Input: part model. Units: mm. Frame: model coordinates. A direction names the side the tool comes from. Round coordinates to 2 decimals unless told otherwise and drop trailing zeros. Loops run counter-clockwise (first coordinate to the right, second up) from the corner with the lowest first, then second, coordinate; pieces in that order, holes last. Notation, with made-up numbers: (83, -15) - (97, -15) arc R21 cw to (97, 19) - close; hole circle Ø3 at (87, 64). An arc over 180 degrees is marked (long way). One line per question, with ' | ' between items. Start each with the question number.
Item 1: Set-up query: faces 1 (the face through (-24.03, -24.06, 39.22)), 2 (the face through (-13, -20, 24.5)), 3 (the face through (-14.24, -24, 5.39)), 4 (the face through (-3, -24, 34.243)), 5 (the face through (-3, -20, 29.5)). Return all of +Z, -Z, +X, -X, +Y, -Y with unobstructed straight access to the full face (end or side cutting, diameter ignored); none if empty.
Item 2: Section A-A, the plane z = 6.5. Return loops of the section in (x, y), plus the area to 3 significant figures.
Item 3: Section B-B, the plane z = 29. Return loops of the section in (x, y), plus the area to 3 significant figures.
Item 4: Draft query along Y for faces 6 (the face through (-20, -24, 0)), 7 (the face through (-23.686, -29.719, 19.975)), 8 (the face through (-23, -28, 29.5)), 9 (the face through (-23, -20, 29.5)). Return one class per face: pulls with the +Y half, pulls with the -Y half, needs draft (parallel to the pull), parting line crosses it, or undercut.
Item 5: First-contact query: pin 1 (0.6 mm diameter, centred on x = -23, y = -28.5, fed in from +Z); pin 2 (1.8 mm diameter, centred on x = -13.23, z = 34.24, fed in from -Y); pin 3 (0.7 mm diameter, centred on x = -3, y = -25, fed in from -Z); pin 4 (5 mm diameter, centred on x = -13.23, z = 6.5, fed in from +Y). Flat tips, straight axial feed; report the tip coordinate or a pass-through.
Item 6: Section D-D, the plane z = 22.5. Return loops of the section in (x, y), plus the area to 3 significant figures.
Item 7: Section C-C, the plane y = -23.5. Give the number of separate pieces and of enclosed holes in the cut face, plus the area to 3 significant figures.
Item 8: Material intervals for line 1 along Y through (x, z) = (-21, 39.5); line 2 along Z through (x, y) = (-12.75, -22); line 3 along Z through (x, y) = (-14, -22.25), sorted ascending.
```python
from build123d import *

# Parameters (mm, degrees)
SKETCH1_W               = 22.054431489
SKETCH1_H               = 12.5
BOSS_EXTRUDE1_DEPTH     = 43
CUT_EXTRUDE1_DEPTH      = 10
CUT_EXTRUDE1_DEPTH_BACK = 15
SKETCH2_R               = 1.5
FILLET3_R               = 2
SKETCH5_R               = 1.5
CUT_EXTRUDE4_DEPTH      = 57.460223181
CUT_EXTRUDE6_DEPTH      = 10
CUT_EXTRUDE6_DEPTH_BACK = 8.5
SKETCH16_W              = 22.254981862
SKETCH16_H              = 2.991460448
SKETCH16_H_2            = 2.962476682
FILLET4_R               = 2
SKETCH17_W              = 18.620112401
SKETCH17_H              = 2.962476682
SKETCH17_H_2            = 2.991460448
CUT_EXTRUDE7_DEPTH      = 5
SKETCH18_W              = 23.815970502
SKETCH18_H              = 0.508634756
SKETCH18_W_2            = 23.819185945
SKETCH18_H_2            = 0.668990904
CUT_EXTRUDE8_DEPTH      = 20


with BuildPart() as part:
    # Sketch1 → Boss-Extrude1 (new body)
    with BuildSketch(Plane.XY):
        with Locations((-13.228930986, -24.070183414)):
            Rectangle(SKETCH1_W, SKETCH1_H)
    extrude(amount=BOSS_EXTRUDE1_DEPTH)

    # Sketch2 → Cut-Extrude1 (cut, two sides: drawn at the far end of the back side and taken through both)
    with BuildSketch(Plane.XZ.offset(30.320183414).offset(-CUT_EXTRUDE1_DEPTH_BACK)):
        with Locations(Location((-13.228930986, 6.5, 0), (0, 0, 90))):
            Circle(SKETCH2_R)
        with Locations(Location((-13.228930986, 34.242856315, 0), (0, 0, 90))):
            Circle(SKETCH2_R)
        with BuildLine():
            Line((-3.452400544, 34.242856315), (-2.201715242, 34.242856315))
            add(Edge.make_bspline(
                [(-24.256146731, 33.845079723), (-30.575526658, 43.607362182), (-11.195866971, 55.012360634), (11.473693948, 42.135391331), (-2.201715242, 34.242856315)],
                knots=[0, 0, 0, 0, 0.486113305, 1, 1, 1, 1], degree=3))
            add(Edge.make_bspline(
                [(-3.757837453, 36.667507789), (-8.059315717, 39.510148032), (-28.688217354, 46.070013084), (-24.256146731, 33.845079723)],
                knots=[0, 0, 0, 0, 1, 1, 1, 1], degree=3))
            ThreePointArc((-3.757837453, 36.667507789), (-3.529060324, 35.464763275), (-3.452400544, 34.242856315))
        make_face()
        with BuildLine():
            Line((-4.478930986, 8.75), (-2.201715242, 8.75))
            add(Edge.make_bspline(
                [(-2.201715242, 8.75), (5.39210746, 3.880294823), (-0.777052631, -4.523329032), (-17.174300591, -10.623347238), (-34.821400648, -0.026005424), (-24.256146731, 8.75)],
                knots=[0, 0, 0, 0, 0.283272691, 0.504244858, 1, 1, 1, 1], degree=3))
            add(Edge.make_bspline(
                [(-23.490579314, 0), (-24.966512963, 4.237786421), (-24.256146731, 8.75)],
                knots=[0, 0, 0, 1, 1, 1], degree=2))
            Line((-23.490579314, 0), (-13.228930986, 0))
            ThreePointArc((-13.228930986, 0), (-7.041746651, 2.562815665), (-4.478930986, 8.75))
        make_face()
    extrude(amount=CUT_EXTRUDE1_DEPTH + CUT_EXTRUDE1_DEPTH_BACK, mode=Mode.SUBTRACT)

    # Fillet3
    # the kernel refuses this fillet: 2 mm, written as the material it takes off along each edge
    with BuildSketch(Plane(origin=(-24.256146731, -17.820183414, -5.498495188), x_dir=(1, 0, 0), z_dir=(0, 0, 1))) as fillet3_piece_1:
        with BuildLine():
            CenterArc((FILLET3_R, -FILLET3_R), FILLET3_R, 90, 90)
            Line((0, -FILLET3_R), (-FILLET3_R * 0.02, -FILLET3_R))
            Line((-FILLET3_R * 0.02, -FILLET3_R), (-FILLET3_R * 0.02, FILLET3_R * 0.02))
            Line((-FILLET3_R * 0.02, FILLET3_R * 0.02), (FILLET3_R, FILLET3_R * 0.02))
            Line((FILLET3_R, FILLET3_R * 0.02), (FILLET3_R, 0))
        make_face()
    extrude(amount=49.579952304, mode=Mode.SUBTRACT)
    with BuildSketch(Plane(origin=(-24.256146731, -30.320183414, -5.498495188), x_dir=(1, 0, 0), z_dir=(0, 0, 1))) as fillet3_piece_2:
        with BuildLine():
            CenterArc((FILLET3_R, FILLET3_R), FILLET3_R, 180, 90)
            Line((0, FILLET3_R), (-FILLET3_R * 0.02, FILLET3_R))
            Line((-FILLET3_R * 0.02, FILLET3_R), (-FILLET3_R * 0.02, -FILLET3_R * 0.02))
            Line((-FILLET3_R * 0.02, -FILLET3_R * 0.02), (FILLET3_R, -FILLET3_R * 0.02))
            Line((FILLET3_R, -FILLET3_R * 0.02), (FILLET3_R, 0))
        make_face()
    extrude(amount=49.579952304, mode=Mode.SUBTRACT)
    with BuildSketch(Plane(origin=(-24.256146731, -17.374523396, 3.001504812), x_dir=(0.16676818592575848, -1.2260366807919533e-15, -0.9859961319209278), z_dir=(0, -1, 0))) as fillet3_piece_3:
        with BuildLine():
            CenterArc((0.168096911, 1.999974157), FILLET3_R, 260.400032587, 9.891234523)
            Line((-0.165439461, 0.027981894), (-0.172110188, -0.011457952))
            Line((-0.172110188, -0.011457952), (-0.006670727, -0.039439845))
            Line((-0.006670727, -0.039439845), (-0.00020343, -0.039999483))
            ThreePointArc((-0.00020343, -0.039999483), (0.089132026, -0.040226606), (0.178467349, -0.039999483))
            Line((0.178467349, -0.039999483), (0.178264007, 0))
        make_face()
    extrude(amount=13.391320036, mode=Mode.SUBTRACT)
    with BuildSketch(Plane(origin=(-24.256146731, -14.845669726, 39.081457115), x_dir=(0.7050638771295608, 0, 0.7091438000624637), z_dir=(0, -1, 0))) as fillet3_piece_4:
        with BuildLine():
            CenterArc((0.853663976, -1.971549871), FILLET3_R, 80.324332734, 54.510372083)
            Line((-0.556463778, -0.553262271), (-0.584666333, -0.524896519))
            Line((-0.584666333, -0.524896519), (-0.028202555, 0.028365752))
            Line((-0.028202555, 0.028365752), (-0.007160044, 0.039353955))
            ThreePointArc((-0.007160044, 0.039353955), (0.595170372, 0.092331415), (1.196528305, 0.039430997))
            Line((1.196528305, 0.039430997), (1.189805475, 0))
        make_face()
    extrude(amount=18.449027376, mode=Mode.SUBTRACT)

    # Sketch5 → Cut-Extrude4 (cut, through all)
    with BuildSketch(Plane.XY):
        with Locations(Location((-18.011106811, -24.070183414, 0), (0, 0, 180))):
            Circle(SKETCH5_R)
        with Locations(Location((-8.446755162, -24.070183414, 0), (0, 0, 180))):
            Circle(SKETCH5_R)
    extrude(amount=CUT_EXTRUDE4_DEPTH, mode=Mode.SUBTRACT)

    # Sketch16 → Cut-Extrude6 (cut, two sides: drawn at the far end of the back side and taken through both)
    with BuildSketch(Plane.XY.offset(38).offset(-CUT_EXTRUDE6_DEPTH_BACK)):
        with Locations((-13.23420775, -20.185246876)):
            Rectangle(SKETCH16_W, SKETCH16_H)
        with Locations((-13.23420775, -27.993084265)):
            Rectangle(SKETCH16_W, SKETCH16_H_2)
    extrude(amount=CUT_EXTRUDE6_DEPTH + CUT_EXTRUDE6_DEPTH_BACK, mode=Mode.SUBTRACT)

    # Fillet4
    fillet4_edges = [part.edges().sort_by_distance(p)[0] for p in [
        (-3.757837453, -18.254850033, 36.667507789),
        (-3.757837453, -24.096411512, 36.667507789),
        (-3.757837453, -29.89725301, 36.667507789),
    ]]
    fillet(fillet4_edges, radius=FILLET4_R)

    # Sketch17 → Cut-Extrude7 (cut)
    with BuildSketch(Plane.XY.offset(29.5)):
        with Locations((-13.043692231, -27.993084265)):
            Rectangle(SKETCH17_W, SKETCH17_H)
        with Locations((-13.043692231, -20.185246876)):
            Rectangle(SKETCH17_W, SKETCH17_H_2)
    extrude(amount=-CUT_EXTRUDE7_DEPTH, mode=Mode.SUBTRACT)

    # Sketch18 → Cut-Extrude8 (cut)
    with BuildSketch(Plane.XY):
        with Locations((-13.361747728, -30.370746627)):
            Rectangle(SKETCH18_W, SKETCH18_H)
        with Locations((-13.36335545, -17.714562357)):
            Rectangle(SKETCH18_W_2, SKETCH18_H_2)
    extrude(amount=CUT_EXTRUDE8_DEPTH, mode=Mode.SUBTRACT)


solid = part.part
```
Return value:
1) face 1: +Z, -X, +Y, -Y | face 2: +Z | face 3: +Y, -Y | face 4: +Z, +X, +Y, -Y | face 5: +Z, +X, -X
2) outline: (-24.26, -28.32) arc R2 ccw to (-23.14, -30.12) - (-14.73, -30.12) - (-14.73, -18.05) - (-23.19, -18.05) arc R2 ccw to (-24.26, -19.82) - close; (-11.73, -30.12) - (-4.77, -30.12) - (-4.77, -18.05) - (-11.73, -18.05) - close; hole circle Ø3 at (-18.01, -24.07); hole circle Ø3 at (-8.45, -24.07) | area: 184 mm2
3) outline: (-24.26, -28.32) arc R2 ccw to (-22.26, -30.32) - (-2.2, -30.32) - (-2.2, -17.82) - (-22.26, -17.82) arc R2 ccw to (-24.26, -19.82) - close; hole (-22.35, -29.47) - (-3.73, -29.47) - (-3.73, -26.51) - (-22.35, -26.51) - close; hole (-22.35, -21.68) - (-3.73, -21.68) - (-3.73, -18.69) - (-22.35, -18.69) - close; hole circle Ø3 at (-18.01, -24.07); hole circle Ø3 at (-8.45, -24.07) | area: 149 mm2
4) face 6: needs draft | face 7: pulls with the -Y half | face 8: undercut | face 9: undercut
5) pin 1: z = 29.5 | pin 2: through | pin 3: z = 8.75 | pin 4: y = -18.05
6) outline: (-24.26, -28.32) arc R2 ccw to (-22.26, -30.32) - (-2.2, -30.32) - (-2.2, -17.82) - (-22.26, -17.82) arc R2 ccw to (-24.26, -19.82) - close; hole circle Ø3 at (-18.01, -24.07); hole circle Ø3 at (-8.45, -24.07) | area: 260 mm2
7) separate pieces: 3 | enclosed holes: 2 | area: 599 mm2
8) line 1: -30.32 to -29.47, -26.51 to -21.68, -18.69 to -17.82 | line 2: 0.01 to 5.08, 7.92 to 32.82, 35.66 to 40.12 | line 3: 0 to 5.21, 7.79 to 32.96, 35.53 to 40.4
